The drawing under review shows one solid part. Ordinate dimensions are in mm from its lowest x, y, z. Round coordinates to 2 decimals unless told otherwise and drop trailing zeros. Order: outer loops, then holes, each group sorted by start corner. A loop starts at its lowest first (then second) coordinate and runs counter-clockwise, first axis right, second up. Notation, with made-up numbers: M 42,41 L 78,41 A5 cw 78,49 Z; hole C -28,28 d1. An arc over 180 degrees is marked long. Use a Markdown table: item, result.
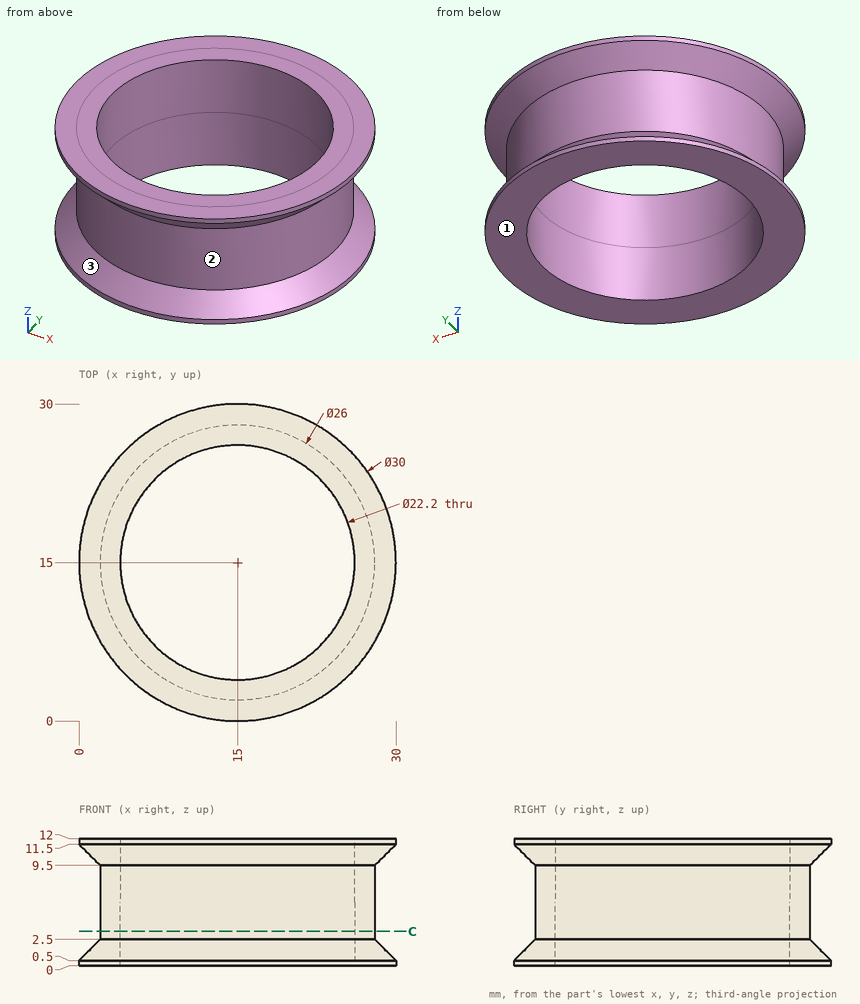
Q1. Draft analysis for pull direction Z (two halves, no side actions). For the marked faces 1, 2 and 3, state which applies: pulls with the +Z half, pulls with the -Z half, needs draft (parallel to the pull), parting line crosses it, or undercut.
Determined:
| item | result |
|---|---|
| face 1 | pulls with the -Z half |
| face 2 | undercut |
| face 3 | undercut |
Q2. Clearance check with flat-ended pins moving along their axes: pin 1 (6 mm diameter, centred on y = 24.5, z = 7.5, fed in from +X); pin 2 (1.5 mm diameter, centred on y = 9.5, z = 4.5, fed in from +X). State where each tip first meets the part, or that it passes through.
Determined:
| item | result |
|---|---|
| pin 1 | stops at x = 26.26 |
| pin 2 | stops at x = 27.1 |
Q3. Wall thickness on line 1 along Y through (x, z) = (15, 8.3); line 2 along X through (y, z) = (20.5, 5.75); line 3 along X through (y, z) = (23, 11) (1 decimal): over which ranges is each line inside the solid? List them lowest first. Write a range as [from, to].
Determined:
| item | result |
|---|---|
| line 1 | y = [2, 3.9], [26.1, 28] |
| line 2 | x = [3.22, 5.36], [24.64, 26.78] |
| line 3 | x = [2.9, 7.3], [22.7, 27.1] |
Q4. Add section C-C (z = 3.25). Write out the cut boundary in (x, y).
Determined:
| item | result |
|---|---|
| outline | C 15,15 d26; hole C 15,15 d22.2 |
